```python
from build123d import *

# Parameters (mm, degrees)
SKETCH1_R                      = 9.4615
EXTRUDE1_DEPTH                 = 3.175
SKETCH2_R                      = 7.8359
EXTRUDE2_DEPTH                 = 9.525
SKETCH3_R                      = 7.4295
CUT_EXTRUDE1_DEPTH             = 0.635
F_8_32_TAPPED_HOLE1_D          = 3.4544
F_8_32_TAPPED_HOLE1_DEPTH      = 12.065
F_1_16_0_0625_DIAMETER_HOLE1_D = 1.5875


with BuildPart() as part:
    # Sketch1 → Extrude1 (new body)
    with BuildSketch(Plane(origin=(0, 0, 0), x_dir=(1, 0, 0), z_dir=(0, 1, 0))):
        with Locations(Location((0, 0, 0), (0, 0, 270))):  # turned: the seam where the file's is
            Circle(SKETCH1_R)
    extrude(amount=EXTRUDE1_DEPTH)

    # Sketch2 → Extrude2 (add)
    with BuildSketch(Plane(origin=(0, 3.175, 0), x_dir=(1, 0, 0), z_dir=(0, 1, 0))):
        with Locations(Location((0, 0, 0), (0, 0, 270))):  # turned: the seam where the file's is
            Circle(SKETCH2_R)
    extrude(amount=EXTRUDE2_DEPTH)

    # Sketch3 → Cut-Extrude1 (cut)
    with BuildSketch(Plane.XZ):
        with Locations(Location((0, 0, 0), (0, 0, 270))):  # turned: the seam where the file's is
            Circle(SKETCH3_R)
    extrude(amount=-CUT_EXTRUDE1_DEPTH, mode=Mode.SUBTRACT)

    # #8-32 Tapped Hole1
    with Locations(Plane.ZX.offset(12.7)):
        with Locations((0, 0)):
            Hole(F_8_32_TAPPED_HOLE1_D / 2, depth=F_8_32_TAPPED_HOLE1_DEPTH)

    # 1/16 (0.0625) Diameter Hole1 (through all)
    with Locations(Plane(origin=(0, 12.7, 0), x_dir=(1, 0, 0), z_dir=(0, 1, 0))):
        with Locations((-4.7625, 0)):
            Hole(F_1_16_0_0625_DIAMETER_HOLE1_D / 2)


solid = part.part
```
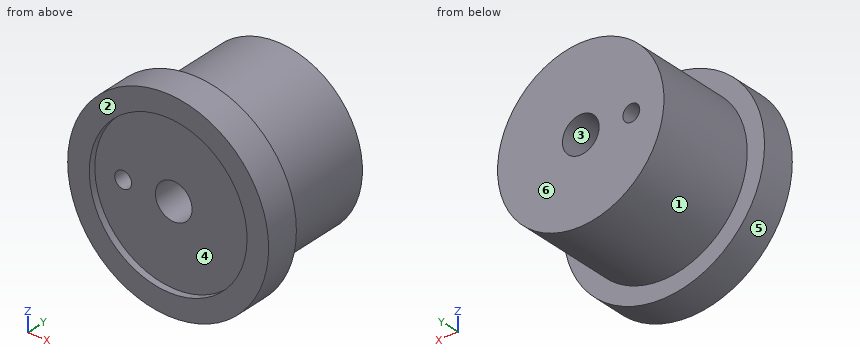
Geometry check sheet. Reference: the model listing, model coordinates, mm. Face numbers are marked on the shaded views. A direction names the side the tool comes from. Give positions to 0.01 mm unless a question says otherwise; leave off trailing zeros. Order: outer loops, then holes, each group sorted by start corner. A loop starts at its lowest first (then second) coordinate and runs counter-clockwise, first axis right, second up. Notation, with made-up numbers: (7, -29.5) - (61, -29.5) arc R33 ccw to (61, 4.5) - close; hole circle Ø11 at (70.5, 15). An arc over 180 degrees is marked (long way). Write item = value, one per line. Start each with the question number.
1) Section check A-A (z = 0). Enter the section's corners in (x, y) (1 decimal).
2) Scan lines: L1, parallel to X at y = 0.3, z = 0; L2, parallel to Y at x = 3.25, z = -2 (3 decimals); L3, parallel to Y at x = -8, z = 2.5 (3 decimals). Record each from-to range of solid material in increasing order.
3) Section check C-C (y = 1.75). Enter the section's corners in (x, z), then the cut area to 3 significant figures.
4) Access from +Z, -Z, +X, -X, +Y, -Y to the whole of each face (thin tool, end or side, straight path). Record for the marked faces 1 and 2.
5) Section check B-B (x = 0). Enter the section's corners in (y, z) (1 decimal).
6) Gauge pin test, flat ends, axial feed: pin 1 Ø4 at (x, z) = (6.5, -0.5) entering from -Y; pin 2 Ø2 at (x, y) = (7, 7) entering from -Z; pin 3 Ø1 at (x, z) = (5.5, 7) entering from +Y (3 decimals); pin 4 Ø1.5 at (y, z) = (7, -7) entering from -X. Record the tip position at first contact, or that the pin passes through.
7) Section check D-D (x = 6.5). Enter the section's corners in (y, z) (3 decimals), then the cut area to 3 significant figures.
8) Draft check along Z on the marked faces 3, 4, 5 and 6. Enter one of: released by +Z, released by -Z, zero draft, split by the parting line, or undercut.
Geometry check:
q1.outline = (-9.5, 0) - (-7.4, 0) - (-7.4, 0.6) - (-5.6, 0.6) - (-5.6, 12.7) - (-7.8, 12.7) - (-7.8, 3.2) - (-9.5, 3.2) - close; (-4, 0.6) - (-1.7, 0.6) - (-1.7, 12.7) - (-4, 12.7) - close; (1.7, 0.6) - (7.4, 0.6) - (7.4, 0) - (9.5, 0) - (9.5, 3.2) - (7.8, 3.2) - (7.8, 12.7) - (1.7, 12.7) - close
q2.L1 = -9.46 to -7.43, 7.43 to 9.46
q2.L2 = 0.635 to 12.7
q2.L3 = 0 to 3.175
q3.outline = circle Ø18.92 at (0, 0); hole circle Ø1.59 at (-4.76, 0); hole circle Ø3.45 at (0, 0)
q3.area = 270 mm2
q4.face_1 = +Y
q4.face_2 = +Z, -Z, +X, -X, -Y
q5.outline = (0, -9.5) - (3.2, -9.5) - (3.2, -7.8) - (12.7, -7.8) - (12.7, -1.7) - (0.6, -1.7) - (0.6, -7.4) - (0, -7.4) - close; (0, 7.4) - (0.6, 7.4) - (0.6, 1.7) - (12.7, 1.7) - (12.7, 7.8) - (3.2, 7.8) - (3.2, 9.5) - (0, 9.5) - close
q6.pin_1 = 0
q6.pin_2 = -5.04
q6.pin_3 = 3.175
q6.pin_4 = -4.73
q7.outline = (0, -6.875) - (3.175, -6.875) - (3.175, -4.376) - (12.7, -4.376) - (12.7, 4.376) - (3.175, 4.376) - (3.175, 6.875) - (0, 6.875) - (0, 3.598) - (0.635, 3.598) - (0.635, -3.598) - (0, -3.598) - close
q7.area = 122 mm2
q8.face_3 = undercut
q8.face_4 = undercut
q8.face_5 = split by the parting line
q8.face_6 = zero draft
